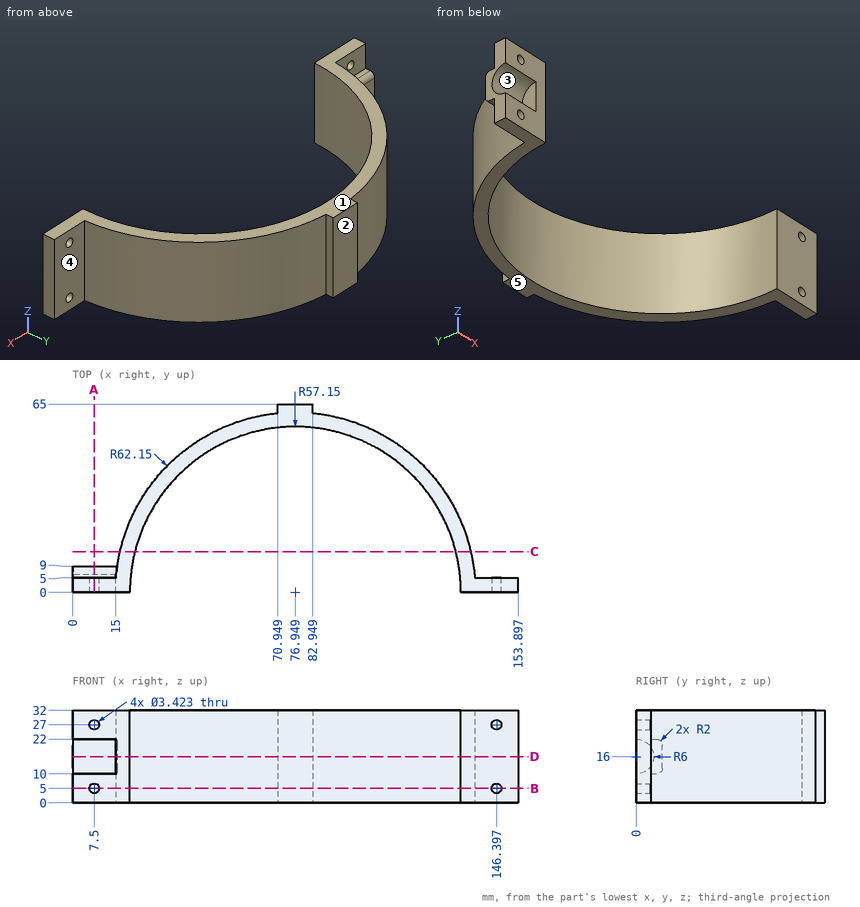
Answer from the drawing. Dimensions are ordinates in mm from the lowest x, y and z of the part. A direction names the side the tool comes from. Round coordinates to 2 decimals unless told otherwise and drop trailing zeros. Write each loop counter-clockwise with the first axis right and the second up, starting at its lowest first coordinate (ties: lowest second). Pieces come first, ordered by that corner, then holes. Notation, with made-up numbers: (-8.75, 1) -> (19.25, 1) arc R19 ccw to (19.25, 30) -> close; hole circle Ø2 at (60.5, 42). An arc over 180 degrees is marked (long way). Answer in a Markdown table with one row per item. Add a question column.
1) Find section B-B, the plane z = 5. State how many separate pieces and enclosed holes the cut face has, and give its area (3 significant figures).
2) Which of the six approach directions +Z, -Z, +X, -X, +Y, -Y give full straight-line access (tool end or side, diameter ignored) to the marked faces 4 and 5?
3) Find section C-C, the plane y = 14. Determine the outline of the cut face in (x, z) (1 decimal), and give its area (3 significant figures).
4) Find section D-D, the plane z = 16. Determine the outline of the cut face in (x, y), and give its area (3 significant figures).
5) Given P1, Ø2.5, axis at y = 64, z = 12, coming from the -X side; P2, Ø12, axis at y = 39.5, z = 20.5, coming from the +X side; P3, Ø8, axis at x = 39, z = 5.5, coming from the -Y side; P4, Ø4.5, axis at x = 7.5, z = 5, coming from the -Y side, each flat-ended and moving along its own axis, determine where each tip first touches the part or whether it passes through.
6) Find section A-A, the plane x = 7.5. Determine the outline of the cut face in (y, z).
7) Determine the mould class of the marked faces 1, 2 and 3 for opening direction Z: pulls with the +Z half, pulls with the -Z half, needs draft (parallel to the pull), parting line crosses it, or undercut.
8) Consider line 1 (Z direction, x = 7.5, y = 2.15); line 2 (Z direction, x = 7, y = 2); line 3 (X direction, y = 10, z = 6.5). Determine where each line is inside the solid, lowest interval first.
Findings below:
| question | item | result |
|---|---|---|
| 1 | separate pieces | 3 |
| 1 | enclosed holes | 0 |
| 1 | area | 1,090 mm² |
| 2 | face 4 | +Z, -Z, +X, +Y |
| 2 | face 5 | -Z, +X, -X, +Y, -Y |
| 3 | outline | (16.4, 0) -> (21.5, 0) -> (21.5, 32) -> (16.4, 32) -> close; (132.4, 0) -> (137.5, 0) -> (137.5, 32) -> (132.4, 32) -> close |
| 3 | area | 329 mm² |
| 4 | outline | (0, 6) -> (15, 6) -> (15, 0) -> (19.8, 0) arc R57.15 cw to (134.1, 0) -> (153.9, 0) -> (153.9, 5) -> (138.9, 5) arc R62.15 ccw to (82.95, 61.86) -> (82.95, 65) -> (70.95, 65) -> (70.95, 61.86) arc R62.15 ccw to (15.45, 9) -> (0, 9) -> close |
| 4 | area | 1,090 mm² |
| 5 | P1 | x = 70.95 |
| 5 | P2 | x = 129.3 |
| 5 | P3 | y = 38.81 |
| 5 | P4 | y = 0 |
| 6 | outline | (0, 0) -> (5, 0) -> (5, 3.29) -> (0, 3.29) -> close; (0, 6.71) -> (5, 6.71) -> (5, 10) -> (7, 10) arc R2 ccw to (9, 12) -> (9, 20) arc R2 ccw to (7, 22) -> (5, 22) -> (5, 25.29) -> (0, 25.29) -> (0, 22) arc R6 cw to (0, 10) -> close; (0, 28.71) -> (5, 28.71) -> (5, 32) -> (0, 32) -> close |
| 7 | face 1 | pulls with the +Z half |
| 7 | face 2 | needs draft |
| 7 | face 3 | undercut |
| 8 | line 1 | 0 to 3.29, 6.71 to 10.4, 21.6 to 25.29, 28.71 to 32 |
| 8 | line 2 | 0 to 3.36, 6.64 to 10.34, 21.66 to 25.36, 28.64 to 32 |
| 8 | line 3 | 15.61 to 20.68, 133.22 to 138.29 |
